```python
from build123d import *

# Parameters (mm, degrees)
BOSS_EXTRUDE1_DEPTH      = 12
BOSS_EXTRUDE1_DEPTH_BACK = 12
SKETCH1_R                = 12
SKETCH2_R                = 9.25
BOSS_EXTRUDE2_DEPTH      = 3
SKETCH3_R                = 3
BOSS_EXTRUDE3_DEPTH      = 1.5
SKETCH4_R                = 0.79375
BOSS_EXTRUDE4_DEPTH      = 7
FILLET1_R                = 0.25
FILLET2_R                = 0.2
SKETCH5_W                = 0.5328248
SKETCH5_H                = 2.687879882
BOSS_EXTRUDE5_DEPTH      = 6.5
SKETCH7_R                = 0.75
CUT_EXTRUDE1_DEPTH       = 35.216099373


with BuildPart() as part:
    # Sketch1 → Boss-Extrude1 (new, two sides: drawn at the far end of the back side and taken through both)
    with BuildSketch(Plane(origin=(0, 0, 0), x_dir=(0, 0, -1), z_dir=(1, 0, 0)).offset(-BOSS_EXTRUDE1_DEPTH_BACK)):
        Circle(SKETCH1_R)
    extrude(amount=BOSS_EXTRUDE1_DEPTH + BOSS_EXTRUDE1_DEPTH_BACK)

    # Sketch2 → Boss-Extrude2 (add)
    with BuildSketch(Plane(origin=(12, 0, 0), x_dir=(0, 0, -1), z_dir=(1, 0, 0))):
        Circle(SKETCH2_R)
    extrude(amount=BOSS_EXTRUDE2_DEPTH)

    # Sketch3 → Boss-Extrude3 (add)
    with BuildSketch(Plane(origin=(15, 0, 0), x_dir=(0, 0, -1), z_dir=(1, 0, 0))):
        Circle(SKETCH3_R)
    extrude(amount=BOSS_EXTRUDE3_DEPTH)

    # Sketch4 → Boss-Extrude4 (add)
    with BuildSketch(Plane(origin=(16.5, 0, 0), x_dir=(0, 0, -1), z_dir=(1, 0, 0))):
        Circle(SKETCH4_R)
    extrude(amount=BOSS_EXTRUDE4_DEPTH)

    # Fillet1
    fillet1_edges = [part.edges().sort_by_distance(p)[0] for p in [
        (12, 0, 12),
        (12, 0, 9.25),
        (15, 0, 9.25),
    ]]
    fillet(fillet1_edges, radius=FILLET1_R)

    # Fillet2
    fillet2_edges = [part.edges().sort_by_distance(p)[0] for p in [
        (16.5, 0, 3),
    ]]
    fillet(fillet2_edges, radius=FILLET2_R)

    # Sketch5 → Boss-Extrude5 (add)
    with BuildSketch(Plane.ZY.offset(12)):
        with Locations((9.5164124, 0)):
            Rectangle(SKETCH5_W, SKETCH5_H)
    boss_extrude5 = extrude(amount=BOSS_EXTRUDE5_DEPTH)

    # Mirror1: Boss-Extrude5 across plane
    add(boss_extrude5.mirror(Plane.XY))

    # Sketch7 → Cut-Extrude1 (cut, through all)
    with BuildSketch(Plane.XY.offset(9.7828248)):
        with Locations((-17, 0)):
            Circle(SKETCH7_R)
    extrude(amount=-CUT_EXTRUDE1_DEPTH, mode=Mode.SUBTRACT)


solid = part.part
```
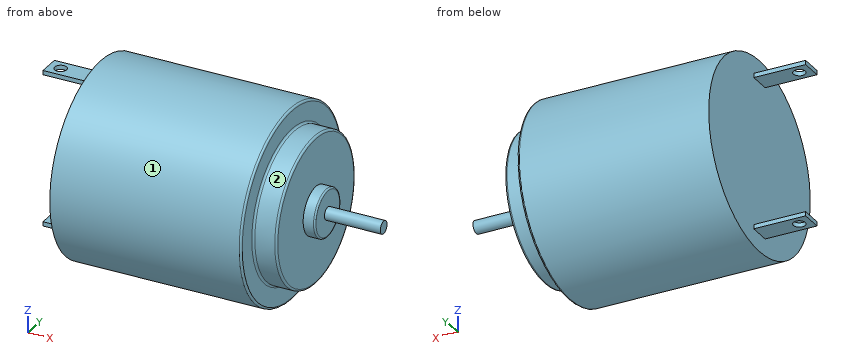
Work out the finished part from the listing and answer in its coordinate system (mm). Face numbers are marked on the shaded views. A direction names the side the tool comes from. Coordinates: 2 decimals unless noted, no trailing zeros. Order: outer loops, then holes, each group sorted by start corner. A loop starts at its lowest first (then second) coordinate and runs counter-clockwise, first axis right, second up. Notation, with made-up numbers: M 78.5,83 L 136.5,83 A15 cw 136.5,87 Z; hole C 33,44 d1. An arc over 180 degrees is marked long. Use CSV: the item, a comma, the result in double quotes.
1) Consider line 1 (Y direction, x = -17, z = 9.65); line 2 (X direction, y = -8.5, z = 7.75); line 3 (X direction, y = 0.75, z = 3). Determine where each line is inside the solid, lowest interval first. Write a range as [from, to].
Worked out:
line 1,"y = [-1.34, -0.75], [0.75, 1.34]"
line 2,"x = [-12, 12]"
line 3,"x = [-12, 15]"
2) For the marked faces 1 and 2, determine the directions among +Z, -Z, +X, -X, +Y, -Y from which every point of the face is accessible in a straight line to the end or side of a thin tool.
Worked out:
face 1,"+X, -X"
face 2,"+X"
3) Flat-ended cylindrical pins translate along their axes: pin 1 Ø1.2 at (x, y) = (-17, 0) entering from +Z; pin 2 Ø7 at (y, z) = (-3, -3.5) entering from -X; pin 3 Ø10 at (x, z) = (-0.5, 5.5) entering from +Y; pin 4 Ø12 at (x, z) = (10.5, -8) entering from -Y. Find the tip coordinate at first contact, or state that the pin passes through.
Worked out:
pin 1,"passes through"
pin 2,"stops at x = -12"
pin 3,"stops at y = 11.99"
pin 4,"stops at y = -11.83"
4) Section C-C on y = 0 is taken. Count the separate pieces of the cut face and the enclosed holes in it, plus the area to 3 significant figures.
Worked out:
separate pieces,"3"
enclosed holes,"0"
area,"657 mm^2"
5) Section A-A on x = -17 is taken. Write down the section's boundary in (y, z).
Worked out:
outline,"M -1.34,-9.78 L -0.75,-9.78 L -0.75,-9.25 L -1.34,-9.25 Z; M -1.34,9.25 L -0.75,9.25 L -0.75,9.78 L -1.34,9.78 Z; M 0.75,-9.78 L 1.34,-9.78 L 1.34,-9.25 L 0.75,-9.25 Z; M 0.75,9.25 L 1.34,9.25 L 1.34,9.78 L 0.75,9.78 Z"
6) Section D-D on x = 6.5 is taken. Write down the section's boundary in (y, z).
Worked out:
outline,"C 0,0 d24"
7) Section B-B on z = 0 is taken. Write down the section's boundary in (x, y), plus the area to 3 significant figures.
Worked out:
outline,"M -12,-12 L 11.75,-12 A0.25 ccw 12,-11.75 L 12,-9.5 A0.25 cw 12.25,-9.25 L 14.75,-9.25 A0.25 ccw 15,-9 L 15,-3 L 16.3,-3 A0.2 ccw 16.5,-2.8 L 16.5,-0.79 L 23.5,-0.79 L 23.5,0.79 L 16.5,0.79 L 16.5,2.8 A0.2 ccw 16.3,3 L 15,3 L 15,9 A0.25 ccw 14.75,9.25 L 12.25,9.25 A0.25 cw 12,9.5 L 12,11.75 A0.25 ccw 11.75,12 L -12,12 Z"
area,"652 mm^2"
